from build123d import *


with BuildPart() as part:
    # Sketch2 → Revolve1 (revolve)
    with BuildSketch(Plane(origin=(0, 0, 0), x_dir=(1, 0, 0), z_dir=(0, 1, 0)), mode=Mode.PRIVATE) as revolve1_sk:
        with BuildLine():
            Line((25.5, 0), (28.5, 0))
            Line((28.5, 0), (28.5, 2.5))
            Line((28.5, 2.5), (26.5, 2.5))
            Line((26.5, 2.5), (16, 7.5))
            Line((16, 7.5), (16, 15.5))
            Line((16, 15.5), (14, 15.5))
            Line((14, 15.5), (14, 16.5))
            Line((14, 16.5), (0, 16.5))
            Line((0, 16.5), (0, 2))
            ThreePointArc((0, 2), (4.366062299, 2.506735229), (8.5, 4))
            Line((8.5, 4), (25.5, 0))
        make_face()
    revolve(revolve1_sk.sketch.rotate(Axis((0, 0, -16.5), (0, 0, 1)), 180), axis=Axis((0, 0, -16.5), (0, 0, 1)))


solid = part.part
Input: part model. Units: mm. Frame: model coordinates. A direction names the side the tool comes from. Coordinates: 2 decimals unless noted, no trailing zeros. Loops run counter-clockwise (first coordinate to the right, second up) from the corner with the lowest first, then second, coordinate; pieces in that order, holes last. Notation, with made-up numbers: (-7.75, -16.75) -> (41.25, -16.75) arc R33 cw to (41.25, 18.25) -> close; hole circle Ø10 at (0, 34.5). An arc over 180 degrees is marked (long way). Write each question's results on one line, items separated by ' | '. Start each with the question number.
Q1. Ray query, line 1 (Z direction, x = -15, y = 22); line 2 (X direction, y = 26, z = -2.25); line 3 (Z direction, x = -8.5, y = -9.5). Return the intervals inside material, ascending. Write a range as from..to.
Q2. Pull-direction query (X, two-part tool) for faces 1 (the conical face through (2.07, 9.34, -3.75)), 2 (the flat face through (0, 0, -16.5)), 3 (the cylindrical face through (3.47, 15.62, -11.56)); classes: released by +X, released by -X, zero draft, split by the parting line, or undercut.
Q3. Pin query (flat end, axial travel): pin 1 (5 mm diameter, centred on x = 3.5, z = -6.5, fed in from +Y); pin 2 (5 mm diameter, centred on y = 7.5, z = -8, fed in from -X); pin 3 (2 mm diameter, centred on x = -15, y = -12, fed in from -Z). Return the tip coordinate at first contact, or that it passes through.
Q4. Reachability of faces 4 (the flat face through (-21, 15, 0)), 5 (the flat face through (0.07, 14.15, -15.5)) from +Z, -Z, +X, -X, +Y, -Y: full face, straight path, thin tool, end or side. Return the list, or none.
Q5. Section D-D, the plane z = -5.75. Return the cut outline in (x, y) (3 decimals), plus the area to 3 significant figures.
Q6. Section A-A, the plane y = 0. Return the cut outline in (x, z) (1 decimal).
Q7. Section C-C, the plane z = -14.75. Return the cut outline in (x, y).
Found:
1) line 1: -2.5..0 | line 2: -11.67..11.67 | line 3: -16.5..-3
2) face 1: undercut | face 2: zero draft | face 3: split by the parting line
3) pin 1: y = 23.1 | pin 2: x = -18.84 | pin 3: z = -6.45
4) face 4: +Z, +X, -X, +Y, -Y | face 5: -Z
5) outline: circle Ø39.35 at (0, 0) | area: 1,220 mm2
6) outline: (-28.5, -2.5) -> (-26.5, -2.5) -> (-16, -7.5) -> (-16, -15.5) -> (-14, -15.5) -> (-14, -16.5) -> (14, -16.5) -> (14, -15.5) -> (16, -15.5) -> (16, -7.5) -> (26.5, -2.5) -> (28.5, -2.5) -> (28.5, 0) -> (25.5, 0) -> (8.5, -4) arc R19.1 ccw to (-8.5, -4) -> (-25.5, 0) -> (-28.5, 0) -> close
7) outline: circle Ø32 at (0, 0)
